```python
from build123d import *

# Parameters (mm, degrees)
ESQUISSE1_W             = 10
ESQUISSE1_H             = 75
BOSS_EXTRU_1_DEPTH      = 10
ESQUISSE2_R             = 1
ESQUISSE2_R_2           = 2
ENL_V_MAT_EXTRU_1_DEPTH = 10
CONG_1_R                = 5
BOSS_EXTRU_2_DEPTH      = 10
CONG_2_R                = 5


with BuildPart() as part:
    # Esquisse1 → Boss.-Extru.1 (new body)
    with BuildSketch(Plane.XY):
        with Locations((5, 37.5)):
            Rectangle(ESQUISSE1_W, ESQUISSE1_H)
    extrude(amount=BOSS_EXTRU_1_DEPTH)

    # Esquisse2 → Enlèv. mat.-Extru.1 (cut)
    with BuildSketch(Plane.XY.offset(10)):
        with Locations((5, 56)):
            Circle(ESQUISSE2_R)
        with Locations((5, 71)):
            Circle(ESQUISSE2_R)
        with Locations((5, 5)):
            Circle(ESQUISSE2_R_2)
    extrude(amount=-ENL_V_MAT_EXTRU_1_DEPTH, mode=Mode.SUBTRACT)

    # Congé1
    cong_1_edges = [part.edges().sort_by_distance(p)[0] for p in [
        (10, 75, 5),
        (0, 75, 5),
    ]]
    fillet(cong_1_edges, radius=CONG_1_R - 0.0001)  # a hair under: the kernel refuses the full size

    # Esquisse3 → Boss.-Extru.2 (add)
    with BuildSketch(Plane.XY.offset(10)):
        with BuildLine():
            Line((0, 0), (-15, 0))
            ThreePointArc((-15, 0), (-0.590052515, 27), (-15, 54))
            Line((-15, 54), (0, 54))
            Line((0, 54), (0, 0))
        make_face()
    extrude(amount=-BOSS_EXTRU_2_DEPTH)

    # Congé2
    cong_2_edges = [part.edges().sort_by_distance(p)[0] for p in [
        (-15, 0, 5),
        (-15, 54, 5),
    ]]
    fillet(cong_2_edges, radius=CONG_2_R)


solid = part.part
```
Design review of the part built by this model. Coordinates are the model's own, in mm. A direction names the side the tool comes from. Round coordinates to 2 decimals unless told otherwise and drop trailing zeros. Order: outer loops, then holes, each group sorted by start corner. A loop starts at its lowest first (then second) coordinate and runs counter-clockwise, first axis right, second up. Notation, with made-up numbers: M 88,-34 L 134,-34 A8 cw 134,-27 Z; hole C -28.75,43 d9. An arc over 180 degrees is marked long. Put each result on its own line as item: value.
Q1. Consider section B-B (x = -4.25). State the section outline as (y, z) points, and give its area (3 significant figures).
Reported:
outline: M 0.24,0 L 12.02,0 L 12.02,10 L 0.24,10 Z; M 41.98,0 L 53.76,0 L 53.76,10 L 41.98,10 Z
area: 236 mm²
Q2. To check wall thickness, follow line 1 (Y direction, x = 5, z = 6.75); line 2 (X direction, y = 65.5, z = 8); line 3 (X direction, y = 71, z = 5.5). State the ranges of each line that lie inside material, in increasing order.
Reported:
line 1: 0 to 3, 7 to 55, 57 to 70, 72 to 75
line 2: 0 to 10
line 3: 0.1 to 4, 6 to 9.9
Q3. Draft analysis for pull direction X (two halves, no side actions). For faces 3 (the face through (5, 70, 5)), 4 (the face through (3, 38, 0)), 5 (the face through (-7.14, 51.34, 4.93)), state which applies: released by +X, released by -X, zero draft, split by the parting line, or undercut.
Reported:
face 3: undercut
face 4: zero draft
face 5: released by -X
Q4. Consider section D-D (y = 28.5). State the section outline as (x, z) points.
Reported:
outline: M -0.62,0 L 10,0 L 10,10 L -0.62,10 Z
Q5. Machinability: for faces 1 (the face through (10, 35, 5)), 2 (the face through (-1, 54, 5)), which of the approach directions +Z, -Z, +X, -X, +Y, -Y give a long, thin tool a straight path to every point of the face, cutting with its end or side? Answer none if there is none.
Reported:
face 1: +Z, -Z, +X, +Y, -Y
face 2: +Z, -Z, -X, +Y
Q6. Insertion check: pin 1 Ø3 at (x, z) = (0, 6.5) entering from +Y; pin 2 Ø4.5 at (x, y) = (5, 5) entering from +Z; pin 3 Ø1.6 at (x, y) = (5, 56) entering from +Z. Each pin has a flat end and moves straight along its axis. Give the tip position at first contact, or say it passes through.
Reported:
pin 1: y = 73.57
pin 2: z = 10
pin 3: through
Q7. Consider section A-A (y = 71). State the section outline as (x, z) points.
Reported:
outline: M 0.1,0 L 4,0 L 4,10 L 0.1,10 Z; M 6,0 L 9.9,0 L 9.9,10 L 6,10 Z
Q8. Consider section C-C (z = 3). State how many separate pieces and enclosed holes the cut face has, and give its area (3 significant figures).
Reported:
separate pieces: 1
enclosed holes: 3
area: 928 mm²
